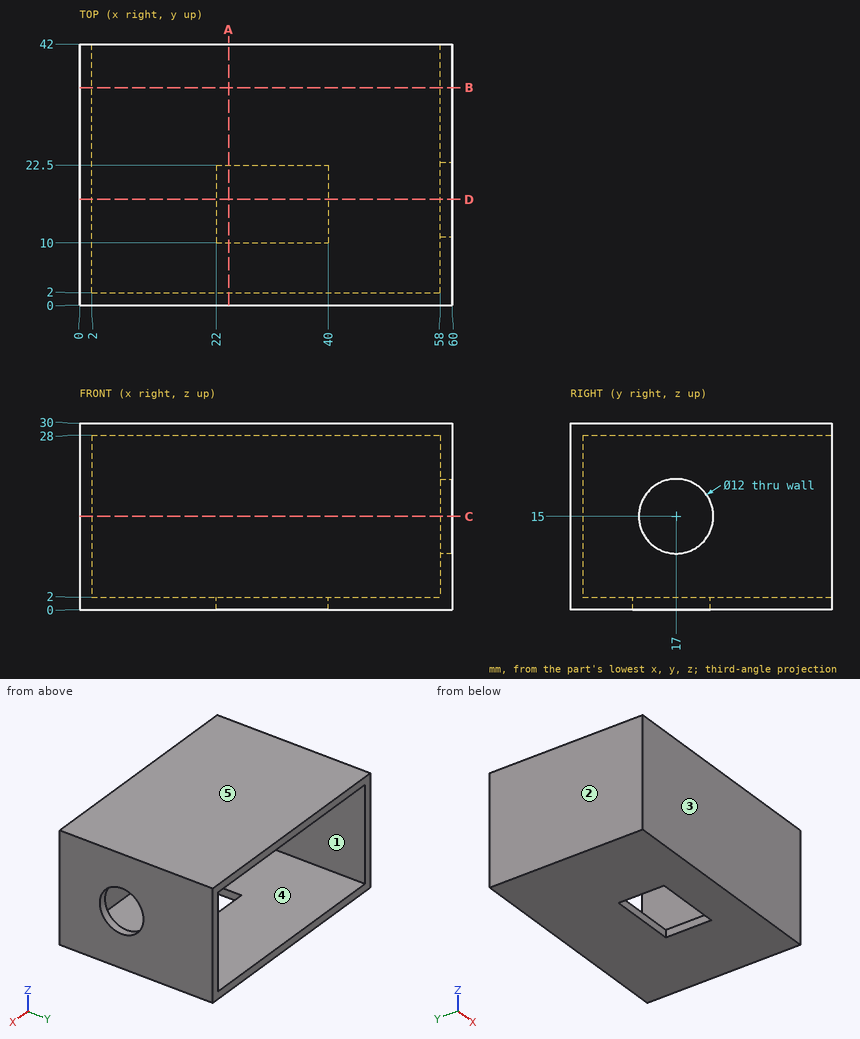
Here's the drawing with two shaded views (mm, measured from the low corner). I have some questions. A direction names the side the tool comes from. Round coordinates to 2 decimals unless told otherwise and drop trailing zeros. Loops run counter-clockwise (first coordinate to the right, second up) from the corner with the lowest first, then second, coordinate; pieces in that order, holes last. Notation, with made-up numbers: M -18,66 L 40,66 A28 ccw 40,91 Z; hole C 17.25,17 d10. An arc over 180 degrees is marked long. Answer as a JSON object with one key per item and string values. Group by question number.
Q1. We'd pull the mould along Z, two halves only. Please class the marked faces 3, 4 and 5: +Z half, -Z half, draft (parallel to the pull), parting line (faces both ways), or undercut.
Q2. Imagine slicing it at D-D, the plane y = 17. Please give me the cut outline in (x, z).
Q3. Imagine slicing it at A-A, the plane x = 24. Please give me the cut outline in (y, z).
Q4. Please list where these lines run through material, in increasing order: L1, parallel to Z at x = 36, y = 27; L2, parallel to X at y = 4.5, z = 26.5; L3, parallel to Y at x = 58.95, z = 15.
Q5. Will these pins go through, and if not, where does the flat tip stop? pin 1 (2 mm diameter, centred on x = 53.5, z = 18, fed in from -Y); pin 2 (8 mm diameter, centred on x = 22, z = 19.5, fed in from +Y); pin 3 (6 mm diameter, centred on x = 28, y = 17.5, fed in from -Z); pin 4 (7 mm diameter, centred on y = 17, z = 15, fed in from +X).
Q6. Imagine slicing it at B-B, the plane y = 35. Please give me the cut outline in (x, z).
Q7. On a 3-axis mill with a long thin cutter (end or side, diameter ignored), from which of +Z, -Z, +X, -X, +Y, -Y can I reach the whole of each face in a straight line? I mean the marked faces 1 and 2. Say none if no direction works.
Q8. Imagine slicing it at C-C, the plane z = 15. Please give me the cut outline in (x, y).
Findings:
{
 "1": {"face 3": "draft", "face 4": "undercut", "face 5": "+Z half"},
 "2": {"outline": "M 0,0 L 22,0 L 22,2 L 2,2 L 2,28 L 58,28 L 58,21 L 60,21 L 60,30 L 0,30 Z; M 40,0 L 60,0 L 60,9 L 58,9 L 58,2 L 40,2 Z"},
 "3": {"outline": "M 0,0 L 10,0 L 10,2 L 2,2 L 2,28 L 42,28 L 42,30 L 0,30 Z; M 22.5,0 L 42,0 L 42,2 L 22.5,2 Z"},
 "4": {"L1": "z = 0 to 2, 28 to 30", "L2": "x = 0 to 2, 58 to 60", "L3": "y = 0 to 11, 23 to 42"},
 "5": {"pin 1": "stops at y = 0", "pin 2": "stops at y = 2", "pin 3": "stops at z = 28", "pin 4": "stops at x = 2"},
 "6": {"outline": "M 0,0 L 60,0 L 60,30 L 0,30 Z; hole M 2,2 L 58,2 L 58,28 L 2,28 Z"},
 "7": {"face 1": "+Y", "face 2": "+Z, -Z, -X, +Y, -Y"},
 "8": {"outline": "M 0,0 L 60,0 L 60,11 L 58,11 L 58,2 L 2,2 L 2,42 L 0,42 Z; M 58,23 L 60,23 L 60,42 L 58,42 Z"}
}
